from build123d import *

# Parameters (mm, degrees)
F1_DEPTH = 127
F2_SIZE  = 19.05
F4_DEPTH = 304.8
F5_R     = 12.7
F6_DEPTH = 38.1


with BuildPart() as f1:
    # F0 (on Front) → F1 (new body)
    with BuildSketch(Plane.XZ):
        Polygon((31.75, 101.6), (0, 101.6), (0, 0), (304.8, 0), (304.8, 101.6), (266.7, 101.6), (266.7, 38.1), (31.75, 38.1), align=None)
    extrude(amount=F1_DEPTH)

    # F2
    f2_edges = [f1.edges().sort_by_distance(p)[0] for p in [
        (0, -63.5, 101.6),
    ]]
    chamfer(f2_edges, length=F2_SIZE)

    # F3 (on Right) → F4 (cut, through all)
    with BuildSketch(Plane.YZ):
        Polygon((-73.250479, 0), (-47.850479, 0), (-47.850479, 16.51), (-28.800479, 16.51), (-28.800479, 29.21), (-47.850479, 29.21), (-47.850479, 38.1), (-73.250479, 38.1), (-73.250479, 29.21), (-92.300479, 29.21), (-92.300479, 16.51), (-73.250479, 16.51), align=None)
    extrude(amount=F4_DEPTH, mode=Mode.SUBTRACT)

    # F5 (on face) → F6 (cut, through all)
    with BuildSketch(Plane.YZ.offset(304.8)):
        with BuildLine():
            Line((-127, 101.6), (-127, 50.8))
            Line((-127, 50.8), (-111.125, 50.8))
            Line((-111.125, 50.8), (-84.593251, 90.349379))
            ThreePointArc((-84.593251, 90.349379), (-63.5, 101.598947), (-42.406749, 90.349379))
            Line((-42.406749, 90.349379), (-15.875, 50.8))
            Line((-15.875, 50.8), (0, 50.8))
            Line((0, 50.8), (0, 101.6))
            Line((0, 101.6), (-127, 101.6))
        make_face()
        with Locations((-63.5, 76.198947)):
            Circle(F5_R)
    extrude(amount=-F6_DEPTH, mode=Mode.SUBTRACT)


solid = f1.part
Could you check a few things on this model? Use its own coordinates, in mm. A direction names the side the tool comes from. Round coordinates to 2 decimals unless told otherwise and drop trailing zeros. Write each loop counter-clockwise with the first axis right and the second up, starting at its lowest first coordinate (ties: lowest second). Pieces come first, ordered by that corner, then holes. Notation, with made-up numbers: (88, 30) -> (96, 30) arc R11 cw to (96, 49) -> close; hole circle Ø9 at (0.5, 64). An arc over 180 degrees is marked (long way). Use a Markdown table: item, result.
1. We'd pull the mould along X, two halves only. Please class faces 6 (the face through (150, -73.25, 8)), 7 (the face through (31.75, -63, 69)), 8 (the face through (0, -63, 42)): +X half, -X half, draft (parallel to the pull), parting line (faces both ways), or undercut.
Answer key:
| item | result |
|---|---|
| face 6 | draft |
| face 7 | undercut |
| face 8 | -X half |
2. If we section it at D-D (z = 72.5): List the corners of the cut face in (x, y) for me.
Answer key:
| item | result |
|---|---|
| outline | (0, -127) -> (31.75, -127) -> (31.75, 0) -> (0, 0) -> close; (266.7, -96.57) -> (304.8, -96.57) -> (304.8, -75.65) -> (266.7, -75.65) -> close; (266.7, -51.35) -> (304.8, -51.35) -> (304.8, -30.43) -> (266.7, -30.43) -> close |
3. For pin 1 Ø12 at (x, z) = (88.5, 45) entering from +Y; pin 2 Ø17.5 at (x, y) = (281.5, -4) entering from +Z; pin 3 Ø21 at (x, y) = (163.5, -38.5) entering from +Z; pin 4 Ø4 at (y, z) = (-60, 84) entering from +X, each with a flat end and sliding along its axis, tell me the tip position at first contact or that it passes through.
Answer key:
| item | result |
|---|---|
| pin 1 | passes through |
| pin 2 | stops at z = 50.8 |
| pin 3 | stops at z = 38.1 |
| pin 4 | stops at x = 31.75 |
4. If we section it at A-A (x = 126): List the corners of the cut face in (y, z) for me, then the cut area to 3 significant figures.
Answer key:
| item | result |
|---|---|
| outline | (-127, 0) -> (-73.25, 0) -> (-73.25, 16.51) -> (-92.3, 16.51) -> (-92.3, 29.21) -> (-73.25, 29.21) -> (-73.25, 38.1) -> (-127, 38.1) -> close; (-47.85, 0) -> (0, 0) -> (0, 38.1) -> (-47.85, 38.1) -> (-47.85, 29.21) -> (-28.8, 29.21) -> (-28.8, 16.51) -> (-47.85, 16.51) -> close |
| area | 3,390 mm^2 |
5. If we section it at C-C (y = -63.5): List the corners of the cut face in (x, z) for me, then the cut area to 3 significant figures.
Answer key:
| item | result |
|---|---|
| outline | (0, 38.1) -> (31.75, 38.1) -> (31.75, 101.6) -> (19.05, 101.6) -> (0, 82.55) -> close; (266.7, 38.1) -> (304.8, 38.1) -> (304.8, 63.5) -> (266.7, 63.5) -> close; (266.7, 88.9) -> (304.8, 88.9) -> (304.8, 101.6) -> (266.7, 101.6) -> close |
| area | 3,290 mm^2 |
6. Which directions (+Z, -Z, +X, -X, +Y, -Y) give clear straight access to the entire face, cutting with the end or side of a thin tool? Please do faces 1 (the face through (151, -100, 38.1)), 2 (the face through (286.017, -63.848, 101.597)), 3 (the face through (150, -73.25, 34)), 4 (the face through (286, -119, 50.8)), 5 (the face through (150, -38, 16.51)).
Answer key:
| item | result |
|---|---|
| face 1 | +Z, +Y, -Y |
| face 2 | +Z, +X |
| face 3 | -Z, +X, -X |
| face 4 | +Z, +X, -Y |
| face 5 | +X, -X |
7. If we section it at B-B (z = 8.5): List the corners of the cut face in (x, y) for me, then the cut area to 3 significant figures.
Answer key:
| item | result |
|---|---|
| outline | (0, -127) -> (304.8, -127) -> (304.8, -73.25) -> (0, -73.25) -> close; (0, -47.85) -> (304.8, -47.85) -> (304.8, 0) -> (0, 0) -> close |
| area | 31,000 mm^2 |
8. Please list where these lines run through material, in increasing order: probe 1 along Z at (x, y) = (259, -46.5); probe 2 along Y at (x, z) = (190, 33); probe 3 along X at (y, z) = (-67.5, 61.5).
Answer key:
| item | result |
|---|---|
| probe 1 | z = 0 to 16.51, 29.21 to 38.1 |
| probe 2 | y = -127 to -73.25, -47.85 to 0 |
| probe 3 | x = 0 to 31.75, 266.7 to 304.8 |
